from build123d import *

# Parameters (mm, degrees)
F0_R     = 1.75
F1_DEPTH = 10
F2_R     = 2.75
F2_R_2   = 1.75
F3_DEPTH = 4
F4_W     = 6
F4_H     = 3
F5_DEPTH = 3
F6_R     = 1
F4_R     = 1.75
F7_DEPTH = 25
F9_DEPTH = 2


with BuildPart() as f1:
    # F0 (on Top) → F1 (new body)
    with BuildSketch(Plane.XY):
        with BuildLine():
            Line((-15.5, -21.15), (15.5, -21.15))
            ThreePointArc((15.5, -21.15), (19.495153, -19.495153), (21.15, -15.5))
            Line((21.15, -15.5), (21.15, 15.5))
            ThreePointArc((21.15, 15.5), (19.495153, 19.495153), (15.5, 21.15))
            Line((15.5, 21.15), (-15.5, 21.15))
            ThreePointArc((-15.5, 21.15), (-19.495153, 19.495153), (-21.15, 15.5))
            Line((-21.15, 15.5), (-21.15, -15.5))
            ThreePointArc((-21.15, -15.5), (-19.495153, -19.495153), (-15.5, -21.15))
        make_face()
        with Locations((-15.5, -15.5)):
            Circle(F0_R, mode=Mode.SUBTRACT)
        with Locations((15.5, -15.5)):
            Circle(F0_R, mode=Mode.SUBTRACT)
        with Locations((-15.5, 15.5)):
            Circle(F0_R, mode=Mode.SUBTRACT)
        with Locations((15.5, 15.5)):
            Circle(F0_R, mode=Mode.SUBTRACT)
    extrude(amount=F1_DEPTH)

    # F2 (on face) → F3 (cut)
    with BuildSketch(Plane(origin=(0, 0, 0), x_dir=(1, 0, 0), z_dir=(0, 0, -1))):
        with Locations((15.5, 15.5)):
            Circle(F2_R)
        with Locations((15.5, 15.5)):
            Circle(F2_R_2, mode=Mode.SUBTRACT)
        with Locations((15.5, -15.5)):
            Circle(F2_R)
        with Locations((15.5, -15.5)):
            Circle(F2_R_2, mode=Mode.SUBTRACT)
        with Locations((-15.5, -15.5)):
            Circle(F2_R)
        with Locations((-15.5, -15.5)):
            Circle(F2_R_2, mode=Mode.SUBTRACT)
        with Locations((-15.5, 15.5)):
            Circle(F2_R)
        with Locations((-15.5, 15.5)):
            Circle(F2_R_2, mode=Mode.SUBTRACT)
    extrude(amount=-F3_DEPTH, mode=Mode.SUBTRACT)

    # F4 (on face) → F5 (join)
    with BuildSketch(Plane(origin=(0, 0, 0), x_dir=(1, 0, 0), z_dir=(0, 0, -1))):
        with Locations((2.85, 6.5)):
            Rectangle(F4_W, F4_H)
        with Locations((-18.15, -6.5)):
            Rectangle(F4_W, F4_H)
        with Locations((-18.15, 6.5)):
            Rectangle(F4_W, F4_H)
        with Locations((2.85, -6.5)):
            Rectangle(F4_W, F4_H)
    extrude(amount=F5_DEPTH)

    # F6
    f6_edges = [f1.edges().sort_by_distance(p)[0] for p in [
        (-21.15, -8, -1.5),
        (-21.15, -5, -1.5),
        (-21.15, 5, -1.5),
        (-15.15, 5, -1.5),
        (-15.15, -8, -1.5),
        (-0.15, -8, -1.5),
        (-0.15, -5, -1.5),
        (-0.15, 5, -1.5),
        (-0.15, 8, -1.5),
        (5.85, -8, -1.5),
        (5.85, 5, -1.5),
        (5.85, -5, -1.5),
        (5.85, 8, -1.5),
        (-15.15, 8, -1.5),
        (-21.15, 8, -1.5),
        (-15.15, -5, -1.5),
    ]]
    fillet(f6_edges, radius=F6_R)

    # F4 (on face) → F7 (cut)
    with BuildSketch(Plane(origin=(0, 0, 0), x_dir=(1, 0, 0), z_dir=(0, 0, -1))):
        with Locations((-7.65, 6.5)):
            Circle(F4_R)
        with Locations((-7.65, -6.5)):
            Circle(F4_R)
    extrude(amount=-F7_DEPTH, mode=Mode.SUBTRACT)

    # F8 (on face) → F9 (cut)
    with BuildSketch(Plane.XY.offset(10)):
        Polygon((-4.9, 4.912287), (-4.9, 8.087713), (-7.65, 9.675426), (-10.4, 8.087713), (-10.4, 4.912287), (-7.65, 3.324574), align=None)
        Polygon((-4.9, -8.087713), (-4.9, -4.912287), (-7.65, -3.324574), (-10.4, -4.912287), (-10.4, -8.087713), (-7.65, -9.675426), align=None)
    extrude(amount=-F9_DEPTH, mode=Mode.SUBTRACT)


solid = f1.part
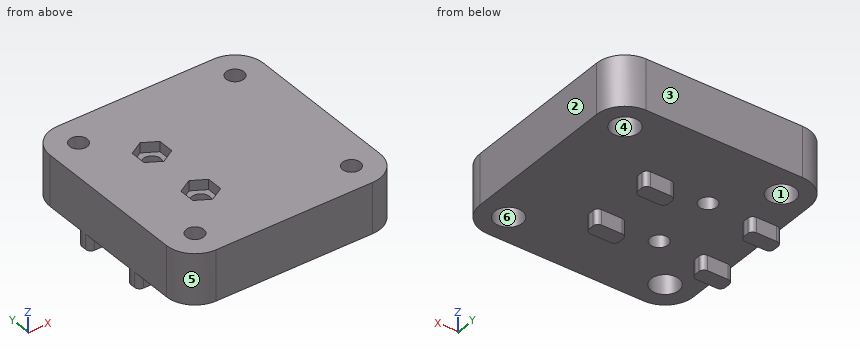
Here's how the part is built. I have some questions about the finished solid (model axes, mm). Face numbers are marked on the shaded views. A direction names the side the tool comes from. Give positions to 0.01 mm unless a question says otherwise; leave off trailing zeros. Order: outer loops, then holes, each group sorted by start corner. A loop starts at its lowest first (then second) coordinate and runs counter-clockwise, first axis right, second up. Notation, with made-up numbers: (45.25, -28.5) -> (58.25, -28.5) arc R24 ccw to (58.25, 3.5) -> close; hole circle Ø11 at (-2.75, -26). An arc over 180 degrees is marked (long way). Use a Markdown table: item, result. Add a question column.
Item 1: Will these pins go through, and if not, where does the flat tip stop? pin 1 (0.5 mm diameter, centred on y = 6.5, z = -2, fed in from +X); pin 2 (2.5 mm diameter, centred on x = -18.5, z = -1, fed in from +Y); pin 3 (3.5 mm diameter, centred on x = 3.5, z = -2, fed in from -Y); pin 4 (6.5 mm diameter, centred on x = -15.5, y = 15.5, fed in from +Z).
Item 2: For the marked faces 5 and 6, which set-ups out of +Z, -Z, +X, -X, +Y, -Y let a thin tool reach every point of the face, with its end or its side?
Item 3: Imagine slicing it at A-A on z = 6. Please give me the cut outline in (x, y).
Item 4: I need wall thicknesses on line 1 (Y direction, x = 15.5, z = 6.7); line 2 (Y direction, x = 15.5, z = 2.1). Which ranges of each line are inside material? Lowest first, please.
Item 5: If we mould it in two halves opening along Y, with no side actions, what happens to the marked faces 1, 2, 3 and 4? For each: pulls with the +Y half, pulls with the -Y half, needs draft (parallel to the pull), parting line crosses it, or undercut.
Item 6: Imagine slicing it at B-B on y = 6.5. Please give me the cut outline in (x, z).
Item 7: Imagine slicing it at C-C on z = -0.5. Give the number of separate pieces and of enclosed holes in the cut face, plus the area to 3 significant figures.
Item 8: Imagine slicing it at D-D on z = 8.5. Please give me the cut outline in (x, y), plus the area to 3 significant figures.
Data:
| question | item | result |
|---|---|---|
| 1 | pin 1 | stops at x = 5.85 |
| 1 | pin 2 | stops at y = 20.68 |
| 1 | pin 3 | stops at y = -8 |
| 1 | pin 4 | stops at z = 10 |
| 2 | face 5 | +Z, -Z, -X, -Y |
| 2 | face 6 | -Z |
| 3 | outline | (-21.15, -15.5) arc R5.65 ccw to (-15.5, -21.15) -> (15.5, -21.15) arc R5.65 ccw to (21.15, -15.5) -> (21.15, 15.5) arc R5.65 ccw to (15.5, 21.15) -> (-15.5, 21.15) arc R5.65 ccw to (-21.15, 15.5) -> close; hole circle Ø3.5 at (-15.5, -15.5); hole circle Ø3.5 at (-15.5, 15.5); hole circle Ø3.5 at (-7.65, -6.5); hole circle Ø3.5 at (-7.65, 6.5); hole circle Ø3.5 at (15.5, -15.5); hole circle Ø3.5 at (15.5, 15.5) |
| 4 | line 1 | y = -21.15 to -17.25, -13.75 to 13.75, 17.25 to 21.15 |
| 4 | line 2 | y = -21.15 to -18.25, -12.75 to 12.75, 18.25 to 21.15 |
| 5 | face 1 | undercut |
| 5 | face 2 | needs draft |
| 5 | face 3 | pulls with the +Y half |
| 5 | face 4 | undercut |
| 6 | outline | (-21.15, -3) -> (-15.15, -3) -> (-15.15, 0) -> (-9.4, 0) -> (-9.4, 8) -> (-10.4, 8) -> (-10.4, 10) -> (-21.15, 10) -> close; (-5.9, 0) -> (-0.15, 0) -> (-0.15, -3) -> (5.85, -3) -> (5.85, 0) -> (21.15, 0) -> (21.15, 10) -> (-4.9, 10) -> (-4.9, 8) -> (-5.9, 8) -> close |
| 7 | separate pieces | 4 |
| 7 | enclosed holes | 0 |
| 7 | area | 68.6 mm² |
| 8 | outline | (-21.15, -15.5) arc R5.65 ccw to (-15.5, -21.15) -> (15.5, -21.15) arc R5.65 ccw to (21.15, -15.5) -> (21.15, 15.5) arc R5.65 ccw to (15.5, 21.15) -> (-15.5, 21.15) arc R5.65 ccw to (-21.15, 15.5) -> close; hole circle Ø3.5 at (-15.5, -15.5); hole circle Ø3.5 at (-15.5, 15.5); hole (-10.4, -8.09) -> (-7.65, -9.68) -> (-4.9, -8.09) -> (-4.9, -4.91) -> (-7.65, -3.32) -> (-10.4, -4.91) -> close; hole (-10.4, 4.91) -> (-7.65, 3.32) -> (-4.9, 4.91) -> (-4.9, 8.09) -> (-7.65, 9.68) -> (-10.4, 8.09) -> close; hole circle Ø3.5 at (15.5, -15.5); hole circle Ø3.5 at (15.5, 15.5) |
| 8 | area | 1,670 mm² |
